Verification items for the finished model (mm, model axes). Face numbers are marked on the shaded views. Coordinates: 2 decimals unless noted, no trailing zeros. Order: outer loops, then holes, each group sorted by start corner. A loop starts at its lowest first (then second) coordinate and runs counter-clockwise, first axis right, second up. Notation, with made-up numbers: (28.25, 60.25) -> (71.25, 60.25) arc R23 ccw to (71.25, 93.25) -> close; hole circle Ø7 at (14, 59.5). An arc over 180 degrees is marked (long way). Write each question's results on one line, items separated by ' | '. Start each with the question number.
(1) Cross-section at B-B on x = 0. Enter the section's corners in (y, z), and give its area (3 significant figures).
(2) Go/stop test with flat-tipped pins: pin 1 (1 mm diameter, centred on y = -6, z = 18.5, fed in from -X); pin 2 (10 mm diameter, centred on y = 7, z = 10.5, fed in from -X); pin 3 (3 mm diameter, centred on x = 8, z = -18, fed in from -Y); pin 4 (2 mm diameter, centred on x = 6.5, y = 0, fed in from -Z). Record where each tip stops, or that it passes through.
(3) Thickness scan on probe 1 along Y at (x, z) = (-6.5, -0.5); probe 2 along Z at (x, y) = (-0.25, -7.25); probe 3 along Z at (x, y) = (-0.75, 3). Record the ranges inside material, lowest first. Write a range as [from, to].
(4) Cross-section at A-A on z = 0. Enter the section's corners in (x, y), and give its area (3 significant figures).
(5) Cross-section at D-D on z = 9.5. Enter the section's corners in (x, y).
(6) Cross-section at C-C on y = 0.75. Enter the section's corners in (x, z), and give its area (3 significant figures).
(7) Draft check along X on the marked faces 1, 2, 3 and 4. Enter one of: +X half, -X half, draft (parallel to the pull), parting line (faces both ways), or undercut.
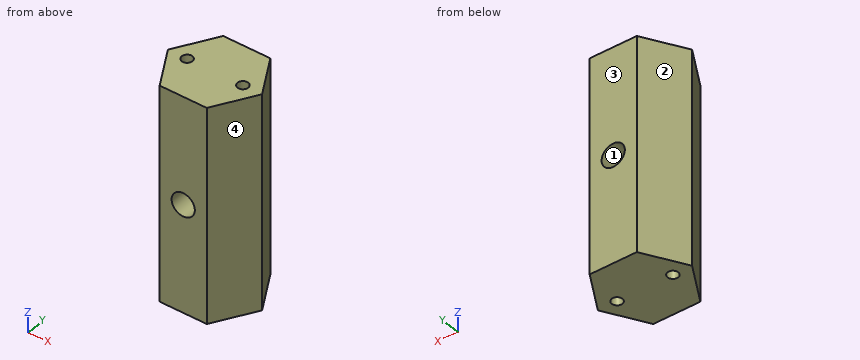
```python
from build123d import *

# Parameters (mm, degrees)
SKETCH1_R                   = 1.25
BOSS_EXTRUDE1_DEPTH         = 25
F_1_4_28_TAPPED_HOLE1_D     = 5.4102
F_1_4_28_TAPPED_HOLE1_DEPTH = 19


with BuildPart() as part:
    # Sketch1 → Boss-Extrude1 (new body, symmetric)
    with BuildSketch(Plane.XY):
        Polygon((-5.484827557, -9.5), (5.484827557, -9.5), (10.969655115, 0), (5.484827557, 9.5), (-5.484827557, 9.5), (-10.969655115, 0), align=None)
        with Locations((-6.5, 0)):
            Circle(SKETCH1_R, mode=Mode.SUBTRACT)
        with Locations((6.5, 0)):
            Circle(SKETCH1_R, mode=Mode.SUBTRACT)
    extrude(amount=BOSS_EXTRUDE1_DEPTH, both=True)

    # 1/4-28 Tapped Hole1
    with Locations(Plane(origin=(0, 9.5, 0), x_dir=(1, 0, 0), z_dir=(0, 1, 0))):
        with Locations((0, 0)):
            Hole(F_1_4_28_TAPPED_HOLE1_D / 2, depth=F_1_4_28_TAPPED_HOLE1_DEPTH)


solid = part.part
```
Results are:
1) outline: (-9.5, -25) -> (9.5, -25) -> (9.5, -2.71) -> (-9.5, -2.71) -> close; (-9.5, 2.71) -> (9.5, 2.71) -> (9.5, 25) -> (-9.5, 25) -> close | area: 847 mm2
2) pin 1: stops at x = -7.79 | pin 2: stops at x = -9.81 | pin 3: stops at y = -7.74 | pin 4: passes through
3) probe 1: y = [-7.74, -1.25], [1.25, 7.74] | probe 2: z = [-25, -2.69], [2.69, 25] | probe 3: z = [-25, -2.6], [2.6, 25]
4) outline: (-10.97, 0) -> (-5.48, -9.5) -> (-2.71, -9.5) -> (-2.71, 9.5) -> (-5.48, 9.5) -> close; (2.71, -9.5) -> (5.48, -9.5) -> (10.97, 0) -> (5.48, 9.5) -> (2.71, 9.5) -> close; hole circle Ø2.5 at (-6.5, 0); hole circle Ø2.5 at (6.5, 0) | area: 200 mm2
5) outline: (-10.97, 0) -> (-5.48, -9.5) -> (5.48, -9.5) -> (10.97, 0) -> (5.48, 9.5) -> (-5.48, 9.5) -> close; hole circle Ø2.5 at (-6.5, 0); hole circle Ø2.5 at (6.5, 0)
6) outline: (-10.54, -25) -> (-7.5, -25) -> (-7.5, 25) -> (-10.54, 25) -> close; (-5.5, -25) -> (5.5, -25) -> (5.5, 25) -> (-5.5, 25) -> close; (7.5, -25) -> (10.54, -25) -> (10.54, 25) -> (7.5, 25) -> close; hole circle Ø5.41 at (0, 0) | area: 831 mm2
7) face 1: undercut | face 2: -X half | face 3: draft | face 4: +X half
